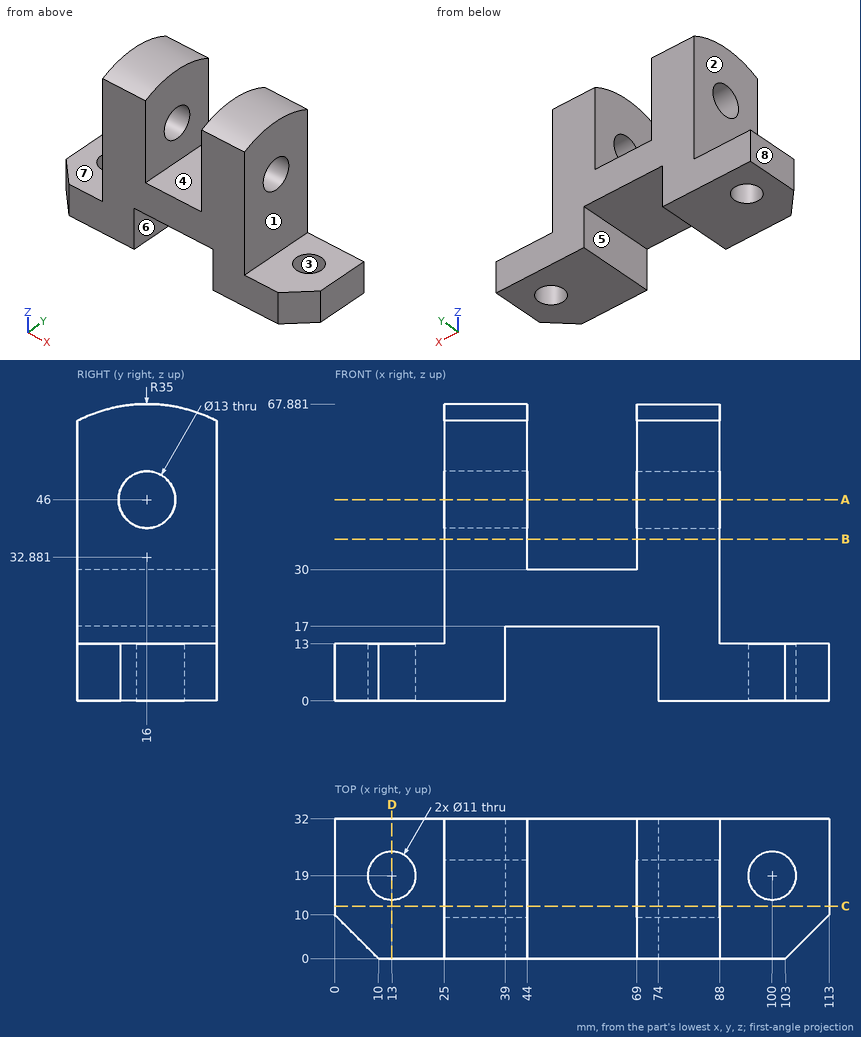
Geometry check sheet. Reference: drawing and pictorial views, mm from the part's lowest x, y, z. A direction names the side the tool comes from. Coordinates: 2 decimals unless noted, no trailing zeros. Order: outer loops, then holes, each group sorted by start corner. A loop starts at its lowest first (then second) coordinate and runs counter-clockwise, first axis right, second up. Notation, with made-up numbers: (-9, 86) - (30, 86) arc R25 ccw to (30, 119) - close; hole circle Ø7 at (28, 32.5). An arc over 180 degrees is marked (long way). Answer in a Markdown table with one row per item. Add a question column.
1) Cross-section at C-C, the plane y = 12. Record the cut outline in (x, z), then the cut area to 3 significant figures.
2) Material ranges on line 1 along Z through (x, y) = (35.5, 16); line 2 along X through (y, z) = (9.5, 37); line 3 along X through (y, z) = (11, 15.5), recorded low to high. Write a range as [from, to].
3) Cross-section at B-B, the plane z = 37. Record the cut outline in (x, y).
4) Set-up check for the marked faces 1, 2, 3, 4 and 5: record each of +Z, -Z, +X, -X, +Y, -Y from which the full face is reachable in a straight line by a thin tool's end or side.
5) Release check for a two-part mould opening along X. For the marked faces 6, 7 and 8 record: +X half, -X half, draft (parallel to the pull), parting line (faces both ways), or undercut.
6) Gauge pin test, flat ends, axial feed: P1, Ø6, axis at y = 7, z = 28.5, coming from the +X side; P2, Ø12.5, axis at x = 12, y = 20, coming from the +Z side; P3, Ø17, axis at y = 16, z = 46, coming from the -X side; P4, Ø6.5, axis at x = 13, y = 19, coming from the +Z side. Record the tip position at first contact, or that the pin passes through.
7) Cross-section at A-A, the plane z = 46. Record the cut outline in (x, y), then the cut area to 3 significant figures.
8) Cross-section at D-D, the plane x = 13. Record the cut outline in (y, z), then the cut area to 3 significant figures.
Check result:
| question | item | result |
|---|---|---|
| 1 | outline | (0, 0) - (39, 0) - (39, 17) - (74, 17) - (74, 0) - (113, 0) - (113, 13) - (88, 13) - (88, 40.88) - (69, 40.88) - (69, 30) - (44, 30) - (44, 40.88) - (25, 40.88) - (25, 13) - (0, 13) - close; (25, 51.12) - (44, 51.12) - (44, 67.65) - (25, 67.65) - close; (69, 51.12) - (88, 51.12) - (88, 67.65) - (69, 67.65) - close |
| 1 | area | 2,990 mm² |
| 2 | line 1 | z = [0, 39.5], [52.5, 67.88] |
| 2 | line 2 | x = [25, 44], [69, 88] |
| 2 | line 3 | x = [25, 39], [74, 88] |
| 3 | outline | (25, 0) - (44, 0) - (44, 32) - (25, 32) - close; (69, 0) - (88, 0) - (88, 32) - (69, 32) - close |
| 4 | face 1 | +Z, +X, +Y, -Y |
| 4 | face 2 | +Z, -X, +Y, -Y |
| 4 | face 3 | +Z, -Z |
| 4 | face 4 | +Z, +Y, -Y |
| 4 | face 5 | -Z, +Y, -Y |
| 5 | face 6 | undercut |
| 5 | face 7 | draft |
| 5 | face 8 | -X half |
| 6 | P1 | stops at x = 88 |
| 6 | P2 | stops at z = 13 |
| 6 | P3 | stops at x = 25 |
| 6 | P4 | passes through |
| 7 | outline | (25, 0) - (44, 0) - (44, 9.5) - (25, 9.5) - close; (25, 22.5) - (44, 22.5) - (44, 32) - (25, 32) - close; (69, 0) - (88, 0) - (88, 9.5) - (69, 9.5) - close; (69, 22.5) - (88, 22.5) - (88, 32) - (69, 32) - close |
| 7 | area | 722 mm² |
| 8 | outline | (0, 0) - (13.5, 0) - (13.5, 13) - (0, 13) - close; (24.5, 0) - (32, 0) - (32, 13) - (24.5, 13) - close |
| 8 | area | 273 mm² |
